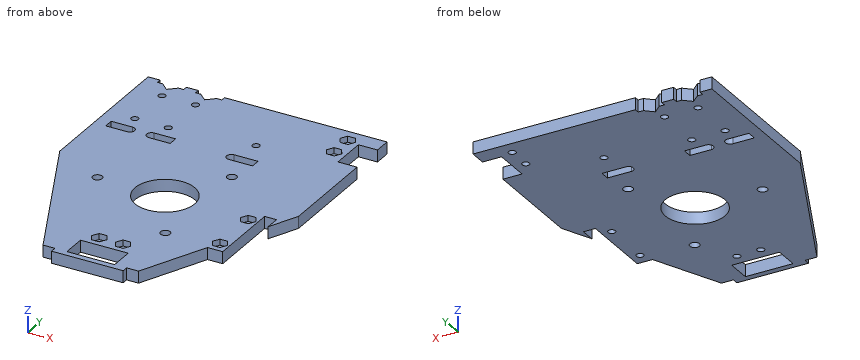
```python
from build123d import *

# Parameters (mm, degrees)
SKETCH_1_W          = 100
SKETCH_1_H          = 130
EXTRUDE_1_DEPTH     = 8
SKETCH_3_W          = 20
SKETCH_3_H          = 10
CUT_EXTRUDE_1_DEPTH = 8
SKETCH_4_R          = 1.5
SKETCH_4_W          = 8
SKETCH_4_H          = 15
CUT_EXTRUDE_2_DEPTH = 9
CUT_EXTRUDE_6_DEPTH = 2.5
SKETCH_10_R         = 12.5
SKETCH_10_W         = 5
SKETCH_10_H         = 30.8
CUT_EXTRUDE_7_DEPTH = 9
EXTRUDE_3_DEPTH     = 8
SKETCH_5_R          = 2
SKETCH_5_R_2        = 1.5
CUT_EXTRUDE_3_DEPTH = 9
SKETCH_11_W         = 30
SKETCH_11_H         = 2.5
EXTRUDE_2_DEPTH     = 8
CUT_EXTRUDE_8_DEPTH = 2.5
SKETCH_15_W         = 100
SKETCH_15_H         = 135
CUT_EXTRUDE_9_DEPTH = 3


with BuildPart() as part:
    # 草图1 → 凸台-拉伸1 (new body)
    with BuildSketch(Plane.XY):
        with Locations((50, 65)):
            Rectangle(SKETCH_1_W, SKETCH_1_H)
    extrude(amount=EXTRUDE_1_DEPTH)

    # 草图3 → 切除-拉伸1 (cut)
    with BuildSketch(Plane.XY.offset(8)):
        with Locations((50, 5)):
            Rectangle(SKETCH_3_W, SKETCH_3_H)
        Polygon((0, 0), (30, 0), (0, 65), align=None)
        Polygon((100, 0), (100, 65), (70, 0), align=None)
    extrude(amount=-CUT_EXTRUDE_1_DEPTH, mode=Mode.SUBTRACT)

    # 草图4 → 切除-拉伸2 (cut, through all)
    with BuildSketch(Plane(origin=(0, 0, 0), x_dir=(-1, 0, 0), z_dir=(0, 0, -1))):
        with Locations((-87, 124)):
            Circle(SKETCH_4_R)
        with Locations((-25.5, 100)):
            Circle(SKETCH_4_R)
        with Locations((-11.5, 100)):
            Circle(SKETCH_4_R)
        with Locations((-11.5, 120)):
            Circle(SKETCH_4_R)
        with Locations((-25.5, 120)):
            Circle(SKETCH_4_R)
        with Locations((-60, 104)):
            Circle(SKETCH_4_R)
        with Locations((-45, 15)):
            Circle(SKETCH_4_R)
        with Locations((-55, 15)):
            Circle(SKETCH_4_R)
        with Locations((-87, 114)):
            Circle(SKETCH_4_R)
        with BuildLine():
            Line((-56.5, 94), (-66.5, 94))
            Line((-66.5, 94), (-66.5, 90))
            Line((-66.5, 90), (-56.5, 90))
            ThreePointArc((-56.5, 90), (-54.5, 92), (-56.5, 94))
        make_face()
        with Locations((-96, 115.5)):
            Rectangle(SKETCH_4_W, SKETCH_4_H)
        with BuildLine():
            Line((-32, 94), (-32, 90))
            Line((-32, 90), (-23, 90))
            ThreePointArc((-23, 90), (-21, 92), (-23, 94))
            Line((-23, 94), (-32, 94))
        make_face()
        with BuildLine():
            Line((-5, 94), (-5, 90))
            Line((-5, 90), (-14, 90))
            ThreePointArc((-14, 90), (-16, 92), (-14, 94))
            Line((-14, 94), (-5, 94))
        make_face()
        Polygon((-10.5, 125), (-13.8, 128), (-16, 128), (-16, 130), (-5, 130), (-5, 128), (-7.2, 128), align=None)
        Polygon((-26.5, 125), (-29.8, 128), (-32, 128), (-32, 130), (-21, 130), (-21, 128), (-23.2, 128), align=None)
    extrude(amount=-CUT_EXTRUDE_2_DEPTH, mode=Mode.SUBTRACT)

    # 草图9 → 切除-拉伸6 (cut)
    with BuildSketch(Plane.XY.offset(8)):
        Polygon((90.175426481, 124), (88.58771324, 126.75), (85.41228676, 126.75), (83.824573519, 124), (85.41228676, 121.25), (88.58771324, 121.25), align=None)
        Polygon((90.175426481, 114), (88.58771324, 116.75), (85.41228676, 116.75), (83.824573519, 114), (85.41228676, 111.25), (88.58771324, 111.25), align=None)
        Polygon((48.175426481, 15), (46.58771324, 17.75), (43.41228676, 17.75), (41.824573519, 15), (43.41228676, 12.25), (46.58771324, 12.25), align=None)
        Polygon((58.175426481, 15), (56.58771324, 17.75), (53.41228676, 17.75), (51.824573519, 15), (53.41228676, 12.25), (56.58771324, 12.25), align=None)
    extrude(amount=-CUT_EXTRUDE_6_DEPTH, mode=Mode.SUBTRACT)

    # 草图10 → 切除-拉伸7 (cut, through all)
    with BuildSketch(Plane.XY.offset(8)):
        with Locations((50, 54.5)):
            Circle(SKETCH_10_R)
        with Locations((91.8, 43.4)):
            Rectangle(SKETCH_10_W, SKETCH_10_H)
    extrude(amount=-CUT_EXTRUDE_7_DEPTH, mode=Mode.SUBTRACT)

    # 草图12 → 凸台-拉伸3 (add)
    with BuildSketch(Plane.XY.offset(8)):
        Polygon((89.3, 41.816666667), (82.923076923, 28), (89.3, 28), align=None)
    extrude(amount=-EXTRUDE_3_DEPTH)

    # 草图5 → 切除-拉伸3 (cut, through all)
    with BuildSketch(Plane.XY.offset(8)):
        with Locations((21.75, 54.5)):
            Circle(SKETCH_5_R)
        with Locations((64.125, 78.965217657)):
            Circle(SKETCH_5_R)
        with Locations((64.125, 30.034782343)):
            Circle(SKETCH_5_R)
        with Locations((85.3, 53.8)):
            Circle(SKETCH_5_R_2)
        with Locations((85.3, 33)):
            Circle(SKETCH_5_R_2)
    extrude(amount=-CUT_EXTRUDE_3_DEPTH, mode=Mode.SUBTRACT)

    # 草图11 → 凸台-拉伸2 (add)
    with BuildSketch(Plane.XY.offset(8)):
        with Locations((50, -1.25)):
            Rectangle(SKETCH_11_W, SKETCH_11_H)
    extrude(amount=-EXTRUDE_2_DEPTH)

    # 草图14 → 切除-拉伸8 (cut)
    with BuildSketch(Plane.XY.offset(8)):
        Polygon((88.475426481, 53.8), (86.88771324, 56.55), (83.71228676, 56.55), (82.124573519, 53.8), (83.71228676, 51.05), (86.88771324, 51.05), align=None)
        Polygon((88.475426481, 33), (86.88771324, 35.75), (83.71228676, 35.75), (82.124573519, 33), (83.71228676, 30.25), (86.88771324, 30.25), align=None)
    extrude(amount=-CUT_EXTRUDE_8_DEPTH, mode=Mode.SUBTRACT)

    # 草图15 → 切除-拉伸9 (cut)
    with BuildSketch(Plane(origin=(0, 0, 0), x_dir=(-1, 0, 0), z_dir=(0, 0, -1))):
        with Locations((-50, 62.5)):
            Rectangle(SKETCH_15_W, SKETCH_15_H)
    extrude(amount=-CUT_EXTRUDE_9_DEPTH, mode=Mode.SUBTRACT)


solid = part.part
```
The model under review builds one solid part; all positions refer to its coordinate system, in mm. Coordinates: 2 decimals unless noted, no trailing zeros. Write each loop counter-clockwise with the first axis right and the second up, starting at its lowest first coordinate (ties: lowest second). Pieces come first, ordered by that corner, then holes.
1) Clearance check with flat-ended pins moving along their axes: pin 1 Ø0.8 at (x, z) = (85.5, 7) entering from -Y; pin 2 Ø0.7 at (x, z) = (22, 6.5) entering from +Y; pin 3 Ø3 at (y, z) = (28.5, 6.5) entering from +X; pin 4 Ø3 at (x, y) = (21.75, 54.5) entering from +Z. State where each tip first meets the part, or that it passes through.
2) We need section A-A on y = 92. State the section outline as (x, z) points.
3) To check wall thickness, follow probe 1 along X at (y, z) = (120, 6.4); probe 2 along Y at (x, z) = (85.3, 4.85); probe 3 along Y at (x, z) = (50, 6.6). State the ranges of each line that lie inside material, in increasing order.
4) We need section B-B on x = 50. State the section outline as (y, z) points.
5) We need section C-C on z = 3.9. Count the separate pieces of the cut face and the enclosed holes in it, then the cut area to 3 significant figures.
Answer list:
1. pin 1: stops at y = 28
1. pin 2: stops at y = 128
1. pin 3: stops at x = 89.3
1. pin 4: passes through
2. outline: (0, 3) - (5, 3) - (5, 8) - (0, 8) - close; (16, 3) - (21, 3) - (21, 8) - (16, 8) - close; (32, 3) - (54.5, 3) - (54.5, 8) - (32, 8) - close; (66.5, 3) - (100, 3) - (100, 8) - (66.5, 8) - close
3. probe 1: x = 0 to 10, 13 to 24, 27 to 92
3. probe 2: y = 28 to 31.5, 34.5 to 52.3, 55.3 to 130
3. probe 3: y = -2.5 to 0, 10 to 42, 67 to 130
4. outline: (-2.5, 3) - (0, 3) - (0, 8) - (-2.5, 8) - close; (10, 3) - (42, 3) - (42, 8) - (10, 8) - close; (67, 3) - (130, 3) - (130, 8) - (67, 8) - close
5. separate pieces: 1
5. enclosed holes: 19
5. area: 9,990 mm2
